```python
from build123d import *

# Parameters (mm, degrees)
SKETCH1_W           = 25
SKETCH1_H           = 24
BOSS_EXTRUDE1_DEPTH = 1
SKETCH2_W           = 8
SKETCH2_H           = 8
BOSS_EXTRUDE2_DEPTH = 5
SKETCH3_W           = 8
SKETCH3_H           = 9
BOSS_EXTRUDE3_DEPTH = 1
SKETCH4_W           = 3
SKETCH4_H           = 2
BOSS_EXTRUDE4_DEPTH = 0.5
CUT_EXTRUDE1_REACH  = 3
SKETCH5_R           = 1.048419625


with BuildPart() as part:
    # Sketch1 → Boss-Extrude1 (new body)
    with BuildSketch(Plane(origin=(0, 0, 0), x_dir=(1, 0, 0), z_dir=(0, 1, 0))):
        Rectangle(SKETCH1_W, SKETCH1_H)
    extrude(amount=BOSS_EXTRUDE1_DEPTH)

    # Sketch2 → Boss-Extrude2 (add)
    with BuildSketch(Plane(origin=(0, 1, 0), x_dir=(1, 0, 0), z_dir=(0, 1, 0))):
        with Locations((0, -3)):
            Rectangle(SKETCH2_W, SKETCH2_H)
    extrude(amount=BOSS_EXTRUDE2_DEPTH)

    # Sketch3 → Boss-Extrude3 (add)
    with BuildSketch(Plane(origin=(0, 1, 0), x_dir=(1, 0, 0), z_dir=(0, 1, 0))):
        with Locations((0, 5.5)):
            Rectangle(SKETCH3_W, SKETCH3_H)
    extrude(amount=BOSS_EXTRUDE3_DEPTH)

    # Sketch4 → Boss-Extrude4 (add)
    with BuildSketch(Plane(origin=(0, 1, 0), x_dir=(1, 0, 0), z_dir=(0, 1, 0))):
        with Locations((8, 8)):
            Rectangle(SKETCH4_W, SKETCH4_H)
    extrude(amount=BOSS_EXTRUDE4_DEPTH)

    # Sketch5 → Cut-Extrude1 (cut, up to next)
    with BuildSketch(Plane(origin=(0, 1, 0), x_dir=(1, 0, 0), z_dir=(0, 1, 0)), mode=Mode.PRIVATE) as cut_extrude1_sk1:
        with Locations((-10.5, 10)):
            Circle(SKETCH5_R)
    cut_extrude1_tool1 = extrude(cut_extrude1_sk1.sketch, amount=-CUT_EXTRUDE1_REACH, mode=Mode.PRIVATE) & part.part
    add(cut_extrude1_tool1.solids().sort_by_distance((-10.5, 1, -10))[0], mode=Mode.SUBTRACT)
    # Sketch5 → Cut-Extrude1 (cut, up to next)
    with BuildSketch(Plane(origin=(0, 1, 0), x_dir=(1, 0, 0), z_dir=(0, 1, 0)), mode=Mode.PRIVATE) as cut_extrude1_sk2:
        with Locations((10.5, 10)):
            Circle(SKETCH5_R)
    cut_extrude1_tool2 = extrude(cut_extrude1_sk2.sketch, amount=-CUT_EXTRUDE1_REACH, mode=Mode.PRIVATE) & part.part
    add(cut_extrude1_tool2.solids().sort_by_distance((10.5, 1, -10))[0], mode=Mode.SUBTRACT)
    # Sketch5 → Cut-Extrude1 (cut, up to next)
    with BuildSketch(Plane(origin=(0, 1, 0), x_dir=(1, 0, 0), z_dir=(0, 1, 0)), mode=Mode.PRIVATE) as cut_extrude1_sk3:
        with Locations((10.5, -2.5)):
            Circle(SKETCH5_R)
    cut_extrude1_tool3 = extrude(cut_extrude1_sk3.sketch, amount=-CUT_EXTRUDE1_REACH, mode=Mode.PRIVATE) & part.part
    add(cut_extrude1_tool3.solids().sort_by_distance((10.5, 1, 2.5))[0], mode=Mode.SUBTRACT)
    # Sketch5 → Cut-Extrude1 (cut, up to next)
    with BuildSketch(Plane(origin=(0, 1, 0), x_dir=(1, 0, 0), z_dir=(0, 1, 0)), mode=Mode.PRIVATE) as cut_extrude1_sk4:
        with Locations((-10.5, -2.5)):
            Circle(SKETCH5_R)
    cut_extrude1_tool4 = extrude(cut_extrude1_sk4.sketch, amount=-CUT_EXTRUDE1_REACH, mode=Mode.PRIVATE) & part.part
    add(cut_extrude1_tool4.solids().sort_by_distance((-10.5, 1, 2.5))[0], mode=Mode.SUBTRACT)


solid = part.part
```
The model under review builds one solid part; all positions refer to its coordinate system, in mm. A direction names the side the tool comes from. Give positions to 0.01 mm unless a question says otherwise; leave off trailing zeros. Write each loop counter-clockwise with the first axis right and the second up, starting at its lowest first coordinate (ties: lowest second). Pieces come first, ordered by that corner, then holes. Notation, with made-up numbers: M 17,-11 L 65,-11 A27 ccw 65,12 Z; hole C -21,47.25 d9. An arc over 180 degrees is marked long. Write each question's results on one line, items separated by ' | '. Start each with the question number.
1. We need section B-B (z = 2.5). Write out the cut boundary in (x, y), and give its area (3 significant figures).
2. We need section D-D (y = 5.15). Write out the cut boundary in (x, z).
3. Insertion check: pin 1 Ø1.5 at (x, z) = (-2.5, -2) entering from -Y; pin 2 Ø0.6 at (x, z) = (8.5, -8) entering from +Y; pin 3 Ø5 at (x, z) = (-9, 7.5) entering from +Y; pin 4 Ø1.9 at (x, z) = (-10.5, 2.5) entering from +Y. Each pin has a flat end and moves straight along its axis. Give the tip position at first contact, or say it passes through.
4. We need section A-A (x = 10.5). Write out the cut boundary in (y, z).
5. We need section C-C (x = -0.75). Write out the cut boundary in (y, z).
6. Mouldability with a two-part tool opening along X and no side actions: class faces 1 (the flat face through (12.5, 0.5, 0.2)), 2 (the flat face through (-0.1, 1.5, -10)), 3 (the cylindrical face through (10.98, 0.51, -9.07)) as released by +X, released by -X, zero draft, split by the parting line, or undercut.
7. For probe 1 along Z at (x, y) = (-10.5, 0.55); probe 2 along X at (y, z) = (0.4, -10); probe 3 along Y at (x, z) = (-6.25, -10.75), list the stretches that pass through material, from the lowest coordinate up. Write a range as [from, to].
8. For faces 4 (the flat face through (8, 1.5, -8)), 5 (the flat face through (0, 4, -1)), 6 (the flat face through (0, 3, 7)), 7 (the flat face through (-4, 3, 2)), list the 3-axis set-ups (+Z, -Z, +X, -X, +Y, -Y) from which the entire face can be reached by the end or side of a thin tool; tool diameter is ignored.
Results found:
1) outline: M -12.5,0 L -11.55,0 L -11.55,1 L -12.5,1 Z; M -9.45,0 L 9.45,0 L 9.45,1 L 4,1 L 4,6 L -4,6 L -4,1 L -9.45,1 Z; M 11.55,0 L 12.5,0 L 12.5,1 L 11.55,1 Z | area: 60.8 mm^2
2) outline: M -4,-1 L 4,-1 L 4,7 L -4,7 Z
3) pin 1: stops at y = 0 | pin 2: stops at y = 1.5 | pin 3: stops at y = 1 | pin 4: passes through
4) outline: M 0,-12 L 1,-12 L 1,-11.05 L 0,-11.05 Z; M 0,-8.95 L 1,-8.95 L 1,1.45 L 0,1.45 Z; M 0,3.55 L 1,3.55 L 1,12 L 0,12 Z
5) outline: M 0,-12 L 1,-12 L 1,-10 L 2,-10 L 2,-1 L 6,-1 L 6,7 L 1,7 L 1,12 L 0,12 Z
6) face 1: released by +X | face 2: zero draft | face 3: undercut
7) probe 1: z = [-12, -11.05], [-8.95, 1.45], [3.55, 12] | probe 2: x = [-12.5, -11.55], [-9.45, 9.45], [11.55, 12.5] | probe 3: y = [0, 1]
8) face 4: +Z, -Z, +X, +Y | face 5: -Z, +X, -X, +Y | face 6: +Z, +X, -X, +Y | face 7: +Z, -Z, -X, +Y
